Source: CAD feature listing. Evaluate the final solid. Frame: model axes, mm. Face numbers are marked on the shaded views. A direction names the side the tool comes from. Give positions to 0.01 mm unless a question says otherwise; leave off trailing zeros. Loops run counter-clockwise (first coordinate to the right, second up) from the corner with the lowest first, then second, coordinate; pieces in that order, holes last. Notation, with made-up numbers: (-4, 81.25) -> (12, 81.25) arc R19 ccw to (12, 102.25) -> close; hole circle Ø2 at (82, 30). An arc over 180 degrees is marked (long way). Put each result on its own line as item: value.
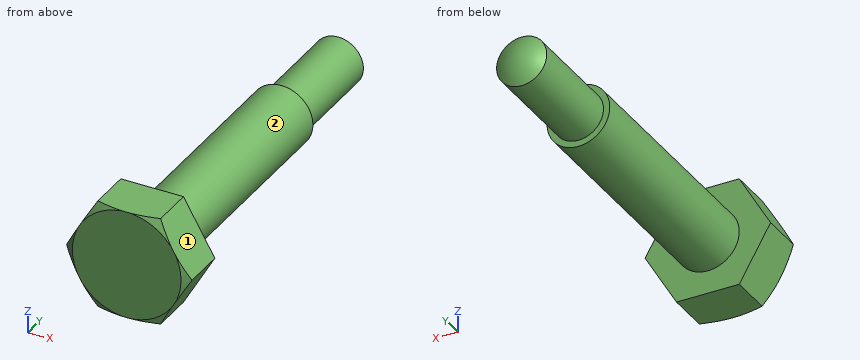
```python
from build123d import *

# Parameters (mm, degrees)
SKETCH1_R           = 7.5
BOSS_EXTRUDE1_DEPTH = 11.2
SKETCH1_3_R         = 7.5
SKETCH1_3_R_2       = 6
BOSS_EXTRUDE2_DEPTH = 68.2
SKETCH1_4_R         = 6
BOSS_EXTRUDE3_DEPTH = 93.2
SKETCH4_OUTSIDE_W   = 338.072
SKETCH4_OUTSIDE_H   = 334.05
SKETCH4_OUTSIDE_R   = 13
CUT_EXTRUDE1_DEPTH  = 82.5
CUT_EXTRUDE1_DRAFT  = -60


with BuildPart() as part:
    # Sketch1 → Boss-Extrude1 (new body)
    with BuildSketch(Plane(origin=(0, 0, 0), x_dir=(1, 0, 0), z_dir=(0, 1, 0))):
        Polygon((15.011106999, 0), (7.505553499, 13), (-7.505553499, 13), (-15.011106999, 0), (-7.505553499, -13), (7.505553499, -13), align=None)
        with Locations(Location((0, 0, 0), (0, 0, 270))):
            Circle(SKETCH1_R, mode=Mode.SUBTRACT)
    extrude(amount=BOSS_EXTRUDE1_DEPTH)

    # Sketch1<3> → Boss-Extrude2 (add)
    with BuildSketch(Plane(origin=(0, 0, 0), x_dir=(1, 0, 0), z_dir=(0, 1, 0))):
        with Locations(Location((0, 0, 0), (0, 0, 270))):
            Circle(SKETCH1_3_R)
        with Locations(Location((0, 0, 0), (0, 0, 270))):
            Circle(SKETCH1_3_R_2, mode=Mode.SUBTRACT)
    extrude(amount=BOSS_EXTRUDE2_DEPTH)

    # Sketch1<4> → Boss-Extrude3 (add)
    with BuildSketch(Plane(origin=(0, 0, 0), x_dir=(1, 0, 0), z_dir=(0, 1, 0))):
        with Locations(Location((0, 0, 0), (0, 0, 270))):
            Circle(SKETCH1_4_R)
    extrude(amount=BOSS_EXTRUDE3_DEPTH)


with BuildPart() as cut_extrude1_tool:
    # Sketch4 outside → Cut-Extrude1 (with draft: the straight prism first)
    with BuildSketch(Plane.XZ):
        Rectangle(SKETCH4_OUTSIDE_W, SKETCH4_OUTSIDE_H)
        Circle(SKETCH4_OUTSIDE_R, mode=Mode.SUBTRACT)
    extrude(amount=-CUT_EXTRUDE1_DEPTH)
    # Cut-Extrude1: the draft: its side faces are tilted about the plane it starts from
    cut_extrude1_sides = [cut_extrude1_tool.faces().sort_by_distance(p)[0] for p in [
        (0, 41.25, -167.025),
        (169.036, 41.25, 0),
        (0, 41.25, 167.025),
        (-169.036, 41.25, 0),
        (-13, 41.25, 0),
    ]]
    draft(cut_extrude1_sides, Plane.XZ, CUT_EXTRUDE1_DRAFT)


with BuildPart() as part_1:
    add(part.part)

    # Cut-Extrude1: cut by cut_extrude1_tool
    add(cut_extrude1_tool.part, mode=Mode.SUBTRACT)

    # Sketch2 → Revolve2 (revolve)
    with BuildSketch(Plane.XY, mode=Mode.PRIVATE) as revolve2_sk:
        with BuildLine():
            Line((-6, 93.2), (0, 93.2))
            Line((0, 93.2), (0, 95.2))
            ThreePointArc((0, 95.2), (-3.16227766, 94.686832981), (-6, 93.2))
        make_face()
    revolve(revolve2_sk.sketch.rotate(Axis((0, 93.2, 0), (0, 1, 0)), 180), axis=Axis((0, 93.2, 0), (0, 1, 0)))


solid = part_1.part
```
(1) Section A-A on y = 6. Return loops of the section in (x, z).
Calculated:
outline: (-15.01, 0) -> (-7.51, -13) -> (7.51, -13) -> (15.01, 0) -> (7.51, 13) -> (-7.51, 13) -> close
(2) Section C-C on y = 29. Return loops of the section in (x, z), then the cut area to 3 significant figures.
Calculated:
outline: circle Ø15 at (0, 0)
area: 177 mm²
(3) Line query: probe 1 along Y at (x, z) = (2.5, -6.75); probe 2 along Y at (x, z) = (3, 11.25); probe 3 along X at (y, z) = (17, 6.25). Output: solid intervals per line, ascending. Write a range as from..to.
Calculated:
probe 1: y = 0..68.2
probe 2: y = 0..11.2
probe 3: x = -4.15..4.15
(4) Section B-B on y = 71. Return loops of the section in (x, z).
Calculated:
outline: circle Ø12 at (0, 0)
(5) Reachability of the marked faces 1 and 2 from +Z, -Z, +X, -X, +Y, -Y: full face, straight path, thin tool, end or side. Return the list, or none.
Calculated:
face 1: +Z, +X, +Y, -Y
face 2: +Y
(6) First-contact query: P1, Ø1, axis at y = 50.5, z = 0, coming from the -X side; P2, Ø4, axis at x = 8, y = 61.5, coming from the -Z side; P3, Ø8, axis at y = 35.5, z = 6.5, coming from the +X side. Flat tips, straight axial feed; report the tip coordinate or a pass-through.
Calculated:
P1: stops at x = -7.5
P2: stops at z = -4.5
P3: stops at x = 7.07
